from build123d import *

# Parameters (mm, degrees)
SKETCH_3_W               = 1500
SKETCH_3_H               = 1500
EXTRUDE_1_DEPTH          = 1500
CUT_EXTRUDE_1_DEPTH      = 2346.207879912
CUT_EXTRUDE_1_DEPTH_BACK = 2346.207879912
SKETCH_4_W               = 1100
SKETCH_4_H               = 1400
CUT_EXTRUDE_2_DEPTH      = 2346.207879912
CUT_EXTRUDE_2_DEPTH_BACK = 2346.207879912
SKETCH_5_W               = 1280
SKETCH_5_H               = 1280
CUT_EXTRUDE_3_DEPTH      = 2346.207879912
CUT_EXTRUDE_3_DEPTH_BACK = 2346.207879912
SKETCH_6_W               = 1290
SKETCH_6_H               = 1280


with BuildPart() as part:
    # 草图3 → 凸台-拉伸1 (new body)
    with BuildSketch(Plane(origin=(0, 0, 0), x_dir=(1, 0, 0), z_dir=(0, 1, 0))):
        with Locations((750, 750)):
            Rectangle(SKETCH_3_W, SKETCH_3_H)
    extrude(amount=EXTRUDE_1_DEPTH)

    # 草图4 → 切除-拉伸1 (cut, two sides: drawn at the far end of the back side and taken through both)
    with BuildSketch(Plane(origin=(1000, 0, 0), x_dir=(0, 0, -1), z_dir=(1, 0, 0)).offset(-CUT_EXTRUDE_1_DEPTH_BACK)):
        with Locations((750, 750)):
            Rectangle(SKETCH_4_W, SKETCH_4_H)
    extrude(amount=CUT_EXTRUDE_1_DEPTH + CUT_EXTRUDE_1_DEPTH_BACK, mode=Mode.SUBTRACT)

    # 草图5 → 切除-拉伸2 (cut, two sides: drawn at the far end of the back side and taken through both)
    with BuildSketch(Plane(origin=(0, 0, -1000), x_dir=(-1, 0, 0), z_dir=(0, 0, -1)).offset(-CUT_EXTRUDE_2_DEPTH_BACK)):
        with Locations((-750, 750)):
            Rectangle(SKETCH_5_W, SKETCH_5_H)
    extrude(amount=CUT_EXTRUDE_2_DEPTH + CUT_EXTRUDE_2_DEPTH_BACK, mode=Mode.SUBTRACT)

    # 草图6 → 切除-拉伸3 (cut, two sides: drawn at the far end of the back side and taken through both)
    with BuildSketch(Plane(origin=(0, 500, 0), x_dir=(-1, 0, 0), z_dir=(0, -1, 0)).offset(-CUT_EXTRUDE_3_DEPTH_BACK)):
        with Locations((-755, 750)):
            Rectangle(SKETCH_6_W, SKETCH_6_H)
    extrude(amount=CUT_EXTRUDE_3_DEPTH + CUT_EXTRUDE_3_DEPTH_BACK, mode=Mode.SUBTRACT)


solid = part.part
Model file for the job. Use its own axes, mm. A direction names the side the tool comes from. Coordinates: 2 decimals unless noted, no trailing zeros. Order: outer loops, then holes, each group sorted by start corner. A loop starts at its lowest first (then second) coordinate and runs counter-clockwise, first axis right, second up. Notation, with made-up numbers: (-24.75, 80.25) -> (-19.75, 80.25) arc R15 cw to (-19.75, 88.25) -> close; hole circle Ø7 at (63.25, 89.25). An arc over 180 degrees is marked (long way). Return JSON: item names as keys, results as strings. Group by question number.
Item 1: Wall check: line 1 along Y through (x, z) = (461.5, -79); line 2 along Y through (x, z) = (71.5, -1044); line 3 along Z through (x, y) = (1421, 611.5). Give the ranges that are in metal, low to high. Write a range as [from, to].
Item 2: Saw through at A-A on z = -293. Write the cut outline in (x, y).
Item 3: Saw through at B-B on y = 760. Write the cut outline in (x, z).
Item 4: Pull direction X, two halves, no side cores. Call faces 5 (the flat face through (806, 87, -1390)), 6 (the flat face through (1406, 740, -1500)), 7 (the flat face through (0, 802, -191)), 8 (the flat face through (759, 1390, -54)): pulls with the +X half, pulls with the -X half, needs draft (parallel to the pull), parting line crosses it, or undercut.
Item 5: Saw through at C-C on x = 174. Write the cut outline in (y, z), then the cut area to 3 significant figures.
Item 6: Tool access for faces 1 (the flat face through (1449, 50, -742)), 2 (the flat face through (1400, 809, -178)), 3 (the flat face through (1406, 0, -760)), 4 (the flat face through (1390, 741, -1444)): list every direction of +Z, -Z, +X, -X, +Y, -Y with a clear straight run to the whole face (end or side of a thin tool).
Values found:
{
 "1": {"line 1": "y = [0, 110], [1390, 1500]", "line 2": "y = [0, 50], [1450, 1500]", "line 3": "z = [-1500, -1300], [-200, 0]"},
 "2": {"outline": "(0, 0) -> (110, 0) -> (110, 50) -> (0, 50) -> close; (0, 1450) -> (110, 1450) -> (110, 1500) -> (0, 1500) -> close; (1400, 0) -> (1500, 0) -> (1500, 50) -> (1400, 50) -> close; (1400, 1450) -> (1500, 1450) -> (1500, 1500) -> (1400, 1500) -> close"},
 "3": {"outline": "(0, -1500) -> (110, -1500) -> (110, -1300) -> (0, -1300) -> close; (0, -200) -> (110, -200) -> (110, 0) -> (0, 0) -> close; (1390, -1500) -> (1500, -1500) -> (1500, -1300) -> (1400, -1300) -> (1400, -1390) -> (1390, -1390) -> close; (1390, -110) -> (1400, -110) -> (1400, -200) -> (1500, -200) -> (1500, 0) -> (1390, 0) -> close"},
 "4": {"face 5": "undercut", "face 6": "needs draft", "face 7": "pulls with the -X half", "face 8": "undercut"},
 "5": {"outline": "(0, -1500) -> (110, -1500) -> (110, -1390) -> (0, -1390) -> close; (0, -110) -> (110, -110) -> (110, 0) -> (0, 0) -> close; (1390, -1500) -> (1500, -1500) -> (1500, -1390) -> (1390, -1390) -> close; (1390, -110) -> (1500, -110) -> (1500, 0) -> (1390, 0) -> close", "area": "48,400 mm2"},
 "6": {"face 1": "+X, -X", "face 2": "+Y, -Y", "face 3": "+Z, -Z, +X, -X, -Y", "face 4": "+Z, -Z"}
}
